The drawing under review shows one solid part. Ordinate dimensions are in mm from its lowest x, y, z. A direction names the side the tool comes from. Round coordinates to 2 decimals unless told otherwise and drop trailing zeros. Loops run counter-clockwise (first coordinate to the right, second up) from the corner with the lowest first, then second, coordinate; pieces in that order, holes last. Notation, with made-up numbers: M -8,88.5 L 3,88.5 A30 cw 3,118.5 Z; hole C 68,-29 d10. An arc over 180 degrees is marked long. Use a Markdown table: item, result.
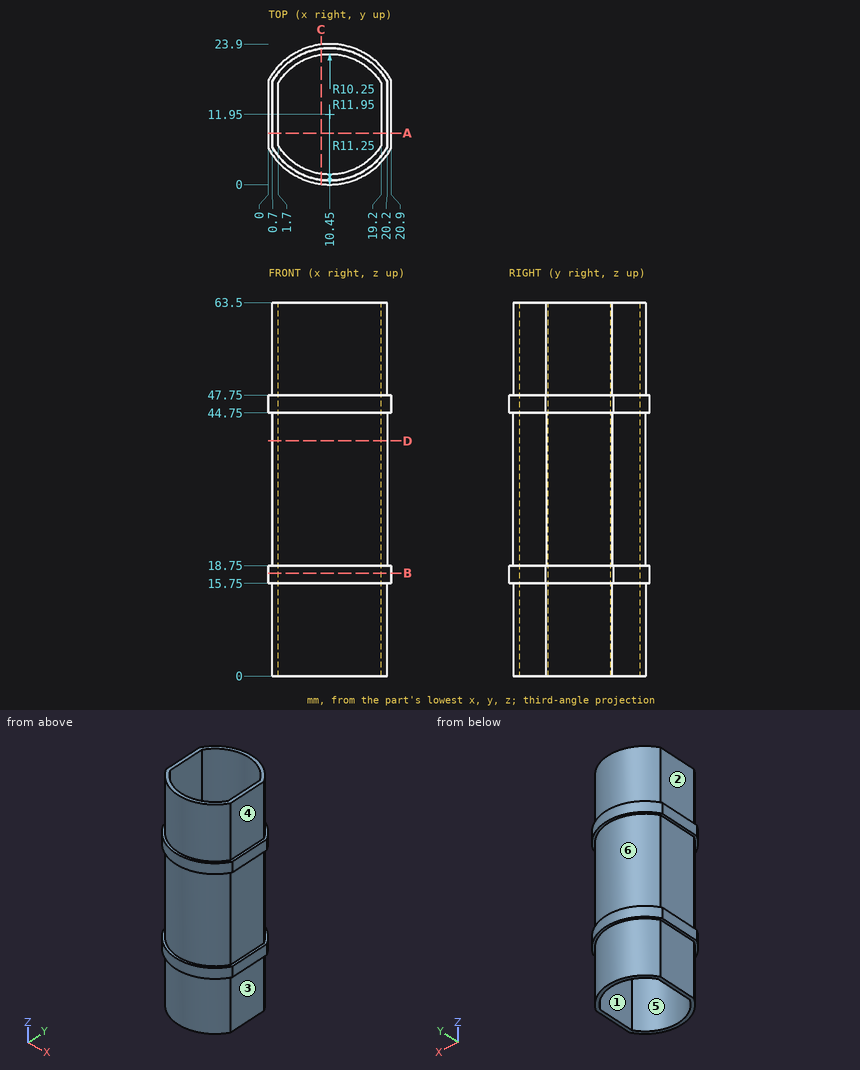
1. Take a section at C-C on x = 9. Give the boundary of the cut face in (y, z).
Check values:
| item | result |
|---|---|
| outline | M 0.09,15.75 L 0.79,15.75 L 0.79,0 L 1.8,0 L 1.8,63.5 L 0.79,63.5 L 0.79,47.75 L 0.09,47.75 L 0.09,44.75 L 0.79,44.75 L 0.79,18.75 L 0.09,18.75 Z; M 22.1,0 L 23.11,0 L 23.11,15.75 L 23.81,15.75 L 23.81,18.75 L 23.11,18.75 L 23.11,44.75 L 23.81,44.75 L 23.81,47.75 L 23.11,47.75 L 23.11,63.5 L 22.1,63.5 Z |
2. Take a section at B-B on z = 17.5. Give the boundary of the cut face in (x, y).
Check values:
| item | result |
|---|---|
| outline | M 0,6.15 A11.95 ccw 20.9,6.15 L 20.9,17.75 A11.95 ccw 0,17.75 Z; hole M 1.7,6.61 A10.25 ccw 19.2,6.61 L 19.2,17.29 A10.25 ccw 1.7,17.29 Z |
3. Insertion check: pin 1 (12 mm diameter, centred on y = 9, z = 17, fed in from -X); pin 2 (5.5 mm diameter, centred on y = 12, z = 30, fed in from +X); pin 3 (6.5 mm diameter, centred on x = 12.5, y = 16.5, fed in from -Z); pin 4 (2 mm diameter, centred on x = 16, z = 25, fed in from +Y). Each pin has a flat end and moves straight along its axis. Give the tip position at first contact, or say it passes through.
Check values:
| item | result |
|---|---|
| pin 1 | stops at x = 0 |
| pin 2 | stops at x = 20.2 |
| pin 3 | passes through |
| pin 4 | stops at y = 22.24 |
4. Take a section at D-D on z = 40. Give the boundary of the cut face in (x, y), and give its area (3 significant figures).
Check values:
| item | result |
|---|---|
| outline | M 0.7,6.34 A11.25 ccw 20.2,6.34 L 20.2,17.56 A11.25 ccw 0.7,17.56 Z; hole M 1.7,6.61 A10.25 ccw 19.2,6.61 L 19.2,17.29 A10.25 ccw 1.7,17.29 Z |
| area | 66.5 mm² |
5. The part is to be moulded in two halves that separate along X. For the marked faces 4, 5 and 6, say which applies: pulls with the +X half, pulls with the -X half, needs draft (parallel to the pull), parting line crosses it, or undercut.
Check values:
| item | result |
|---|---|
| face 4 | pulls with the +X half |
| face 5 | undercut |
| face 6 | parting line crosses it |
6. Machinability: for the marked faces 1, 2 and 3, which of the approach directions +Z, -Z, +X, -X, +Y, -Y give a long, thin tool a straight path to every point of the face, cutting with its end or side? Answer none if there is none.
Check values:
| item | result |
|---|---|
| face 1 | +Z, -Z |
| face 2 | +Z, -X, +Y, -Y |
| face 3 | -Z, +X, +Y, -Y |
7. Wall thickness on line 1 along X through (y, z) = (14.25, 32.5); line 2 along Z through (x, y) = (4.75, 1.75); line 3 along Y through (x, z) = (2.5, 49): over which ranges is each line inside the solid? List them lowest first. Write a range as from..to.
Check values:
| item | result |
|---|---|
| line 1 | x = 0.7..1.7, 19.2..20.2 |
| line 2 | z = 15.75..18.75, 44.75..47.75 |
| line 3 | y = 3.99..5.48, 18.42..19.91 |
8. Take a section at A-A on y = 8.75. Give the boundary of the cut face in (x, z), and give its area (3 significant figures).
Check values:
| item | result |
|---|---|
| outline | M 0,15.75 L 0.7,15.75 L 0.7,0 L 1.7,0 L 1.7,63.5 L 0.7,63.5 L 0.7,47.75 L 0,47.75 L 0,44.75 L 0.7,44.75 L 0.7,18.75 L 0,18.75 Z; M 19.2,0 L 20.2,0 L 20.2,15.75 L 20.9,15.75 L 20.9,18.75 L 20.2,18.75 L 20.2,44.75 L 20.9,44.75 L 20.9,47.75 L 20.2,47.75 L 20.2,63.5 L 19.2,63.5 Z |
| area | 135 mm² |
